```python
from build123d import *

# Parameters (mm, degrees)
F1_DEPTH    = 10
F3_R        = 44.99999
F4_W        = 31
F4_H        = 42
F5_DEPTH    = 11
F6_R        = 5.25
F7_DEPTH    = 7
F9_D        = 10
F9_DEPTH    = 10.001
F10_D       = 6.5
F10_ON_F6_D = 6.5
F11_W       = 31
F11_H       = 2.5
F12_DEPTH   = 1.7
F13_W       = 2.5
F13_H       = 14.5
F14_DEPTH   = 1.7
F16_DEPTH   = 25


# Not quite as in the source:
# - a fillet or chamfer is up to 0.001 mm smaller than in the source, because OpenCascade refuses the exact size


with BuildPart() as f1:
    # F0 (on Top) → F1 (new body)
    with BuildSketch(Plane.XY):
        with BuildLine():
            Line((-45, 70), (-45, 0))
            ThreePointArc((-45, 0), (0, -45), (45, 0))
            Line((45, 0), (45, 70))
            Line((45, 70), (-45, 70))
        make_face()
    extrude(amount=F1_DEPTH)

    # F3 (radius 45 in the source; OpenCascade refuses exactly that, so slightly less here)
    f3_edges = [f1.edges().sort_by_distance(p)[0] for p in [
        (-45, 70, 5),
        (45, 70, 5),
    ]]
    fillet(f3_edges, radius=F3_R)

    # F4 (on face) → F5 (cut)
    with BuildSketch(Plane.XY.offset(10)):
        with Locations((2.9, 3.3)):
            Rectangle(F4_W, F4_H)
    extrude(amount=-F5_DEPTH, mode=Mode.SUBTRACT)

    # F6 (on face) → F7 (join)
    with BuildSketch(Plane(origin=(0, 0, 0), x_dir=(1, 0, 0), z_dir=(0, 0, -1))):
        with Locations((0, -60)):
            Circle(F6_R)
        with Locations((-20, 30)):
            Circle(F6_R)
        with Locations((20, 30)):
            Circle(F6_R)
    extrude(amount=F7_DEPTH)

    # F9 (through all, one way)
    with BuildSketch(Plane(origin=(0, 0, 0), x_dir=(1, 0, 0), z_dir=(0, 0, -1))):
        with Locations((-20, 30), (20, 30), (0, -60)):
            Circle(F9_D / 2)
    extrude(amount=-F9_DEPTH, mode=Mode.SUBTRACT)

    # F10 (through all)
    with Locations(Plane.XY):
        with Locations((20, -30), (0, 60)):
            Hole(F10_D / 2)

    # F10 on F6 (through all)
    with Locations(Plane.XY):
        with Locations((-20, -30)):
            Hole(F10_ON_F6_D / 2)

    # F11 (on face) → F12 (join)
    with BuildSketch(Plane(origin=(0, 0, 0), x_dir=(1, 0, 0), z_dir=(0, 0, -1))):
        with Locations((2.9, -25.55)):
            Rectangle(F11_W, F11_H)
    extrude(amount=F12_DEPTH)

    # F13 (on face) → F14 (join)
    with BuildSketch(Plane(origin=(0, 0, 0), x_dir=(1, 0, 0), z_dir=(0, 0, -1))):
        with Locations((-38.25, 6.55)):
            Rectangle(F13_W, F13_H)
    extrude(amount=F14_DEPTH)

    # F15 (on face) → F16 (cut)
    with BuildSketch(Plane(origin=(-39.5, 0, 0), x_dir=(0, -1, 0), z_dir=(-1, 0, 0))):
        Polygon((13, -1), (13, 0), (0, 0), (0, -1), (2.55, -1), (2.55, -1.7), (10.55, -1.7), (10.55, -1), align=None)
    extrude(amount=-F16_DEPTH, mode=Mode.SUBTRACT)


solid = f1.part
```
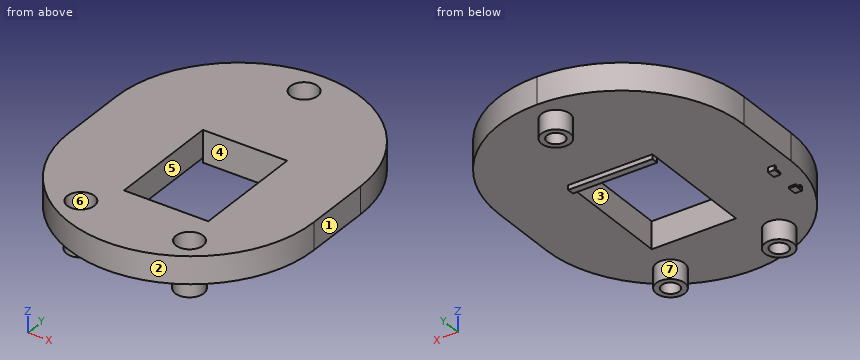
Verification items for the finished model (mm, model axes). Face numbers are marked on the shaded views. A direction names the side the tool comes from. Round coordinates to 2 decimals unless told otherwise and drop trailing zeros. Write each loop counter-clockwise with the first axis right and the second up, starting at its lowest first coordinate (ties: lowest second). Pieces come first, ordered by that corner, then holes.
1. Draft check along Y on the marked faces 1, 2, 3 and 4. Enter one of: +Y half, -Y half, draft (parallel to the pull), parting line (faces both ways), or undercut.
2. Section check D-D on y = -30. Enter the section's corners in (x, z).
3. Scan lines: L1, parallel to Y at x = 0, z = -2.75; L2, parallel to Y at x = 0.5, z = 8.5; L3, parallel to Y at x = -20, z = -4.25. Record each from-to range of solid material in increasing order.
4. Gauge pin test, flat ends, axial feed: P1, Ø0.8, axis at x = -38, z = -1.5, coming from the -Y side; P2, Ø3, axis at y = -12, z = -1, coming from the +X side; P3, Ø5, axis at x = -20, y = -30, coming from the -Z side; P4, Ø3, axis at x = -22, y = -32, coming from the +Z side. Record the tip position at first contact, or that the pin passes through.
5. Access from +Z, -Z, +X, -X, +Y, -Y to the whole of each face (thin tool, end or side, straight path). Record for the marked faces 5, 6 and 7.
6. Section check B-B on x = -11. Enter the section's corners in (y, z).
7. Section check A-A on z = 5.75. State how many separate pieces and enclosed holes the cut face has, plus the area to 3 significant figures.
8. Section check C-C on y = 60. Enter the section's corners in (x, z).
Answer:
1. face 1: draft
1. face 2: -Y half
1. face 3: undercut
1. face 4: undercut
2. outline: (-33.54, 0) - (-25.25, 0) - (-25.25, -7) - (-23.25, -7) - (-23.25, 0) - (-25, 0) - (-25, 10) - (-33.54, 10) - close; (-16.75, -7) - (-14.75, -7) - (-14.75, 0) - (14.75, 0) - (14.75, -7) - (16.75, -7) - (16.75, 0) - (15, 0) - (15, 10) - (-15, 10) - (-15, 0) - (-16.75, 0) - close; (23.25, -7) - (25.25, -7) - (25.25, 0) - (33.54, 0) - (33.54, 10) - (25, 10) - (25, 0) - (23.25, 0) - close
3. L1: y = 54.75 to 56.75, 63.25 to 65.25
3. L2: y = -45 to -17.7, 24.3 to 55.03, 64.97 to 70
3. L3: y = -35.25 to -33.25, -26.75 to -24.75
4. P1: stops at y = -13.8
4. P2: stops at x = 43.66
4. P3: passes through
4. P4: stops at z = 0
5. face 5: +Z, -Z
5. face 6: +Z
5. face 7: -Z
6. outline: (-43.63, 0) - (-17.7, 0) - (-17.7, 10) - (-43.63, 10) - close; (24.3, -1.7) - (26.8, -1.7) - (26.8, 0) - (68.63, 0) - (68.63, 10) - (24.3, 10) - close
7. separate pieces: 1
7. enclosed holes: 4
7. area: 7,070 mm2
8. outline: (-28.28, 0) - (-5.25, 0) - (-5.25, -7) - (-3.25, -7) - (-3.25, 0) - (-5, 0) - (-5, 10) - (-28.28, 10) - close; (3.25, -7) - (5.25, -7) - (5.25, 0) - (28.28, 0) - (28.28, 10) - (5, 10) - (5, 0) - (3.25, 0) - close
